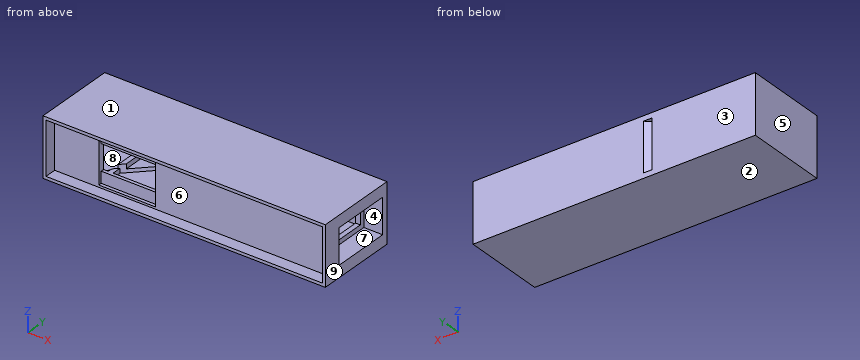
Autodesk Inventor part; units mm, degrees
ref_plane "YZ Plane" through (0, 0, 0) normal (1, 0, 0) x (0, 1, 0)
ref_plane "XZ Plane" through (0, 0, 0) normal (0, 1, 0) x (-1, 0, 0)
ref_plane "XY Plane" through (0, 0, 0) normal (0, 0, 1) x (1, 0, 0)
sketch "Sketch1" plane through (0, 0, 0) normal (0, 1, 0) x (-1, 0, 0)
  line L0 (0, 0) -> (152.4, 0)
  line L1 (152.4, 0) -> (152.4, -31.75)
  line L2 (152.4, -31.75) -> (0, -31.75)
  line L3 (0, -31.75) -> (0, 0)
  line L4 (127, -8.89) -> (96.52, -8.89)
  line L5 (96.52, -8.89) -> (96.52, -22.86)
  line L6 (96.52, -22.86) -> (127, -22.86)
  line L7 (127, -22.86) -> (127, -8.89)
  line L8 (117.2368, -8.89) -> (117.2368, 0)
  line L9 (117.2368, -22.86) -> (117.2368, -31.75)
  dimension "d0" = 152.4
  dimension "d1" = 31.75
  dimension "d2" = 30.48
  dimension "d3" = 13.97
  dimension "d4" = 25.4
extrude "Extrusion1" add sketch "Sketch1" along normal blind 1.778 contours L0 L8 L4 L5 L6 L9 L2 L3 | L0 L1 L2 L9 L6 L7 L4 L8
sketch "Sketch2" plane through (0, 0, 0) normal (0, -1, 0) x (1, 0, 0)
  line L0 (-152.4, 0) -> (0, 0)
  line L1 (0, 0) -> (0, -31.75)
  line L2 (-152.4, 0) -> (0, 0)
  line L3 (0, 0) -> (0, -31.75)
  line L4 (0, -31.75) -> (-152.4, -31.75)
  line L5 (-152.4, -31.75) -> (-152.4, 0)
  line L6 (-127, -2.7348) -> (-96.52, -2.7348)
  line L7 (-96.52, -2.7348) -> (-96.52, -29.0152)
  line L8 (-96.52, -29.0152) -> (-127, -29.0152)
  line L9 (-127, -29.0152) -> (-127, -2.7348)
  line L10 (-127, -8.89) -> (-127, -22.86)
  line L11 (-103.8171, -2.7348) -> (-103.8171, 0)
  line L12 (-104.7941, -29.0152) -> (-104.7941, -31.75)
  line L13 (0, -31.75) -> (-152.4, -31.75)
  dimension "d7" = 30.48
  dimension "d8" = 0
extrude "Extrusion2" add sketch "Sketch2" along normal blind 1.778 contours L0 L11 L6 L9 L8 L12 L4 L5 | L0 L1 L4 L12 L8 L7 L6 L11
sketch "Sketch3" plane through (0, -1.778, 0) normal (0, -1, 0) x (1, 0, 0)
  line L0 (-152.4, 0) -> (0, 0)
  line L1 (0, -31.75) -> (-152.4, -31.75)
  line L2 (-152.4, 0) -> (0, 0)
  line L3 (0, 0) -> (0, -31.75)
  line L4 (0, -31.75) -> (-152.4, -31.75)
  line L5 (-152.4, -31.75) -> (-152.4, 0)
  line L6 (-1.5875, -30.1625) -> (-1.5875, -1.5875)
  line L7 (-1.5875, -1.5875) -> (-150.8125, -1.5875)
  line L8 (-150.8125, -1.5875) -> (-150.8125, -30.1625)
  line L9 (-150.8125, -30.1625) -> (-1.5875, -30.1625)
  dimension "d11" = 1.5875
extrude "Extrusion3" add sketch "Sketch3" along normal blind 6.35
sketch "Sketch4" plane through (0, 1.778, 0) normal (0, 1, 0) x (1, 0, 0)
  line L0 (-152.4, 0) -> (0, 0)
  line L1 (-152.4, 31.75) -> (-152.4, 0)
  line L2 (0, 0) -> (-152.4, 0)
  line L3 (-152.4, 0) -> (-152.4, 31.75)
  line L4 (-152.4, 31.75) -> (0, 31.75)
  line L5 (-6.35, 25.4) -> (-146.05, 25.4)
  line L6 (-146.05, 25.4) -> (-146.05, 6.35)
  line L7 (-146.05, 6.35) -> (-6.35, 6.35)
  line L8 (-13.5859, 25.4) -> (0, 25.4)
  line L9 (0, 0) -> (0, 31.75)
  line L10 (-13.5859, 6.35) -> (0, 6.35)
  line L11 (0, 31.75) -> (0, 25.4)
  line L12 (0, 6.35) -> (0, 0)
  line L13 (-127, 22.86) -> (-96.52, 22.86)
  line L14 (-96.52, 22.86) -> (-93.98, 22.86)
  line L15 (-93.98, 22.86) -> (-93.98, 25.4)
  line L16 (-93.98, 25.4) -> (-96.52, 25.4)
  line L17 (-96.52, 25.4) -> (-96.52, 22.86)
  line L18 (-96.52, 2.7348) -> (-96.52, 29.0152)
  line L19 (-96.52, 6.35) -> (-93.98, 6.35)
  line L20 (-93.98, 6.35) -> (-93.98, 8.89)
  line L21 (-93.98, 8.89) -> (-96.52, 8.89)
  line L22 (-96.52, 8.89) -> (-96.52, 6.35)
  line L23 (-121.92, 25.4) -> (-124.46, 25.4)
  line L24 (-124.46, 25.4) -> (-124.46, 22.86)
  line L25 (-124.46, 22.86) -> (-121.92, 22.86)
  line L26 (-121.92, 22.86) -> (-121.92, 25.4)
  line L27 (-121.92, 6.35) -> (-124.46, 6.35)
  line L28 (-124.46, 6.35) -> (-124.46, 8.89)
  line L29 (-124.46, 8.89) -> (-121.92, 8.89)
  line L30 (-121.92, 8.89) -> (-121.92, 6.35)
  line L31 (-68.58, 25.4) -> (-66.04, 25.4)
  line L32 (-66.04, 25.4) -> (-66.04, 22.86)
  line L33 (-66.04, 22.86) -> (-68.58, 22.86)
  line L34 (-68.58, 22.86) -> (-68.58, 25.4)
  line L35 (-68.58, 6.35) -> (-66.04, 6.35)
  line L36 (-66.04, 6.35) -> (-66.04, 8.89)
  line L37 (-66.04, 8.89) -> (-68.58, 8.89)
  line L38 (-68.58, 8.89) -> (-68.58, 6.35)
  line L39 (-40.64, 6.35) -> (-38.1, 6.35)
  line L40 (-38.1, 6.35) -> (-38.1, 8.89)
  line L41 (-38.1, 8.89) -> (-40.64, 8.89)
  line L42 (-40.64, 8.89) -> (-40.64, 6.35)
  line L43 (-40.64, 25.4) -> (-38.1, 25.4)
  line L44 (-38.1, 25.4) -> (-38.1, 22.86)
  line L45 (-38.1, 22.86) -> (-40.64, 22.86)
  line L46 (-40.64, 22.86) -> (-40.64, 25.4)
  line L47 (-12.7, 25.4) -> (-10.16, 25.4)
  line L48 (-10.16, 25.4) -> (-10.16, 22.86)
  line L49 (-10.16, 22.86) -> (-12.7, 22.86)
  line L50 (-12.7, 22.86) -> (-12.7, 25.4)
  line L51 (-12.7, 6.35) -> (-10.16, 6.35)
  line L52 (-10.16, 6.35) -> (-10.16, 8.89)
  line L53 (-10.16, 8.89) -> (-12.7, 8.89)
  line L54 (-12.7, 8.89) -> (-12.7, 6.35)
  point P0 (-121.92, 7.62)
  point P1 (-96.52, 7.62)
  point P2 (-93.98, 24.13)
  point P3 (-68.58, 24.13)
  point P4 (-40.64, 24.13)
  point P5 (-66.04, 24.13)
  point P6 (-12.7, 24.13)
  point P7 (-38.1, 24.13)
  point P8 (-6.35, 6.35)
  dimension "d14" = 6.35
  dimension "d15" = 2.54
  dimension "d16" = 2.54
  dimension "d17" = 2.54
  dimension "d18" = 2.54
  dimension "d19" = 2.54
  dimension "d20" = 2.54
  dimension "d21" = 25.4
  dimension "d22" = 2.54
  dimension "d23" = 2.54
  dimension "d24" = 2.54
  dimension "d25" = 2.54
  dimension "d26" = 2.54
  dimension "d27" = 2.54
  dimension "d28" = 2.54
  dimension "d29" = 2.54
  dimension "d30" = 2.54
  dimension "d31" = 2.54
  dimension "d32" = 2.54
  dimension "d33" = 2.54
  dimension "d34" = 25.4
  dimension "d35" = 25.4
  dimension "d36" = 25.4
extrude "Extrusion4" add sketch "Sketch4" along normal blind 31.75 contours L1 L4 L9 L8 L5 L6 L7 L10 L0 | L7 L54 L53 L52 | L48 L49 L50 L5 | L7 L42 L41 L40 | L44 L45 L46 L5 | L7 L38 L37 L36 | L32 L33 L34 L5 | L7 L18 L21 L20 | L15 L14 L17 L5 | L7 L28 L29 L30 | L26 L13 L24 L5
sketch "Sketch5" plane through (-93.98, 1.778, -8.89) normal (0, 0, -1) x (-1, 0, 0)
  line L0 (2.54, 31.75) -> (0, 31.75)
  line L1 (0, 31.75) -> (0, 29.21)
  line L2 (0, 29.21) -> (2.54, 29.21)
  line L3 (2.54, 29.21) -> (2.54, 31.75)
  line L4 (30.48, 31.75) -> (27.94, 31.75)
  line L5 (30.48, 0) -> (30.48, 31.75)
  line L6 (27.94, 31.75) -> (30.48, 31.75)
  line L7 (30.48, 31.75) -> (30.48, 29.21)
  line L8 (30.48, 29.21) -> (27.94, 29.21)
  line L9 (27.94, 29.21) -> (27.94, 31.75)
  line L10 (-27.94, 0) -> (-27.94, 31.75)
  line L11 (-25.4, 0) -> (-25.4, 31.75)
  line L12 (-27.94, 29.21) -> (-25.4, 29.21)
  line L13 (-25.4, 29.21) -> (-25.4, 31.75)
  line L14 (-25.4, 31.75) -> (-27.94, 31.75)
  line L15 (-27.94, 31.75) -> (-27.94, 29.21)
  line L16 (-93.98, 31.75) -> (58.42, 31.75)
  line L17 (-27.94, 31.75) -> (-25.4, 31.75)
  line L18 (-25.4, 31.75) -> (-25.4, 29.21)
  line L19 (-25.4, 29.21) -> (-27.94, 29.21)
  line L20 (-27.94, 29.21) -> (-27.94, 31.75)
  line L21 (-53.34, 31.75) -> (-55.88, 31.75)
  line L22 (-55.88, 31.75) -> (-55.88, 29.21)
  line L23 (-55.88, 29.21) -> (-53.34, 29.21)
  line L24 (-53.34, 29.21) -> (-53.34, 31.75)
  line L25 (-81.28, 31.75) -> (-83.82, 31.75)
  line L26 (-83.82, 31.75) -> (-83.82, 29.21)
  line L27 (-83.82, 29.21) -> (-81.28, 29.21)
  line L28 (-81.28, 29.21) -> (-81.28, 31.75)
  line L29 (30.48, 31.75) -> (52.07, 31.75)
  line L30 (30.48, 31.75) -> (27.94, 31.75)
  line L31 (27.94, 31.75) -> (27.94, 29.21)
  line L32 (27.94, 29.21) -> (30.48, 29.21)
  line L33 (30.48, 29.21) -> (30.48, 31.75)
  point P0 (-93.98, -1.778)
  point P1 (0, 30.48)
  point P2 (-25.4, 30.48)
  point P3 (-27.94, 30.48)
  point P4 (-53.34, 30.48)
  point P5 (-81.28, 30.48)
  point P6 (-55.88, 30.48)
  point P7 (27.94, 30.48)
  point P8 (2.54, 30.48)
  dimension "d39" = 2.54
  dimension "d40" = 2.54
  dimension "d41" = 2.54
  dimension "d42" = 2.54
  dimension "d43" = 2.54
  dimension "d44" = 2.54
  dimension "d45" = 25.4
  dimension "d46" = 25.4
  dimension "d47" = 2.54
  dimension "d48" = 2.54
  dimension "d49" = 25.4
  dimension "d50" = 2.54
  dimension "d51" = 2.54
  dimension "d52" = 25.4
extrude "Extrusion5" add sketch "Sketch5" along normal up to next
sketch "Sketch6" plane through (0, 33.528, 0) normal (0, 1, 0) x (1, 0, 0)
  line L0 (-152.4, 31.75) -> (-152.4, 0)
  line L1 (0, 31.75) -> (-152.4, 31.75)
  line L2 (-152.4, 0) -> (0, 0)
  line L3 (0, 0) -> (0, 31.75)
  line L4 (0, 31.75) -> (-152.4, 31.75)
  line L5 (-152.4, 31.75) -> (-152.4, 0)
extrude "Extrusion6" add sketch "Sketch6" along normal blind 3.175
ref_plane "Work Plane1" through (-127, 1.778, -8.89) normal (0.7071, -0.7071, 0) x (0, 0, -1)
sketch "Sketch7" plane through (-127, 1.778, -8.89) normal (0.7071, -0.7071, 0) x (0, 0, -1)
  line L0 (20.1252, -1.2572) -> (20.1252, 20.2954)
  line L1 (20.1252, 0) -> (-6.1552, 0)
  line L2 (-6.1552, 0) -> (-6.1552, 127)
  line L3 (-6.1552, 127) -> (20.1252, 127)
  line L4 (20.1252, 127) -> (20.1252, 0)
  line L5 (0, 0) -> (13.97, 0)
  point P0 (-8.89, 88.5453)
  point P1 (20.1252, 20.2954)
  dimension "d58" = 0
  dimension "d59" = 127
extrude "Extrusion7" cut sketch "Sketch7" against normal blind 3.175
sketch "Sketch8" plane through (0, 1.778, 0) normal (0, 1, 0) x (1, 0, 0)
  line L0 (63.8737, 171.7375) -> (-193.0507, 171.7375)
  line L1 (-193.0507, 171.7375) -> (-193.0507, -76.4775)
  line L2 (-193.0507, -76.4775) -> (63.8737, -76.4775)
  line L3 (63.8737, -76.4775) -> (63.8737, 171.7375)
  point P0 (0, 0)
properties part number "Full Print"
Design review of the part built by this model. Coordinates are the model's own, in mm. Face numbers are marked on the shaded views. A direction names the side the tool comes from. Coordinates: 2 decimals unless noted, no trailing zeros. Loops run counter-clockwise (first coordinate to the right, second up) from the corner with the lowest first, then second, coordinate; pieces in that order, holes last. Notation, with made-up numbers: (19, 26.5) - (71, 26.5) arc R25 cw to (71, 65.5) - close; hole circle Ø5 at (-28.75, 30.5). An arc over 180 degrees is marked (long way). Use CSV: the item, a comma, the result in double quotes. Start each with the question number.
1. Add section C-C on z = -27.5. Give the boundary of the cut face in (x, y).
2. For the marked faces 5, 6, 7, 8 and 9, list the 3-axis set-ups (+Z, -Z, +X, -X, +Y, -Y) from which the entire face can be reached by the end or side of a thin tool; tool diameter is ignored.
3. Clearance check with flat-ended pins moving along their axes: pin 1 (1 mm diameter, centred on x = -79.5, z = -5, fed in from -Y); pin 2 (3 mm diameter, centred on y = 18.5, z = -16.5, fed in from +X); pin 3 (15 mm diameter, centred on y = 25.5, z = -17, fed in from +X). State where each tip first meets the part, or that it passes through.
4. Add section A-A on x = -133.5. Give the boundary of the cut face in (y, z).
5. Mouldability with a two-part tool opening along Z and no side actions: class the marked faces 1, 2, 3 and 4 as released by +Z, released by -Z, zero draft, split by the parting line, or undercut.
6. Add section B-B on y = -3.5. Give the boundary of the cut face in (x, z).
7. To check wall thickness, follow probe 1 along X at (y, z) = (18, -8); probe 2 along Z at (x, y) = (-108, 21); probe 3 along Y at (x, z) = (-82.5, -23). State the ranges of each line that lie inside material, in increasing order.
Resolved:
1,outline,"(-152.4, -8.13) - (-150.81, -8.13) - (-150.81, -1.78) - (-127, -1.78) - (-127, 0) - (-96.52, 0) - (-96.52, -1.78) - (-1.59, -1.78) - (-1.59, -8.13) - (0, -8.13) - (0, 36.7) - (-92.07, 36.7) - (-127, 1.78) - (-129.25, 4.02) - (-96.57, 36.7) - (-152.4, 36.7) - close"
2,face 5,"+Z, -Z, -X, +Y, -Y"
2,face 6,"-Y"
2,face 7,"+X"
2,face 8,"none"
2,face 9,"+Z, -Z, +X, +Y, -Y"
3,pin 1,"y = -1.78"
3,pin 2,"x = -146.05"
3,pin 3,"x = -10.16"
4,outline,"(-8.13, -31.75) - (36.7, -31.75) - (36.7, 0) - (-8.13, 0) - (-8.13, -1.59) - (-1.78, -1.59) - (-1.78, -30.16) - (-8.13, -30.16) - close; hole (1.78, -25.4) - (33.53, -25.4) - (33.53, -6.35) - (1.78, -6.35) - close"
5,face 1,"released by +Z"
5,face 2,"released by -Z"
5,face 3,"zero draft"
5,face 4,"undercut"
6,outline,"(-152.4, -31.75) - (0, -31.75) - (0, 0) - (-152.4, 0) - close; hole (-150.81, -30.16) - (-1.59, -30.16) - (-1.59, -1.59) - (-150.81, -1.59) - close"
7,probe 1,"-152.4 to -146.05, -124.46 to -121.92, -96.52 to -93.98, -68.58 to -66.04, -40.64 to -38.1, -12.7 to -10.16"
7,probe 2,"-31.75 to -29.02, -2.73 to 0"
7,probe 3,"-1.78 to 1.78, 33.53 to 36.7"
